Input: part model. Units: mm. Frame: model coordinates. A direction names the side the tool comes from. Coordinates: 2 decimals unless noted, no trailing zeros. Order: outer loops, then holes, each group sorted by start corner. A loop starts at its lowest first (then second) coordinate and runs counter-clockwise, first axis right, second up.
Autodesk Inventor part; units mm, degrees
ref_plane "Work Plane2" through (-37, -48, -28.5) normal (0, 0, 1) x (1, 0, 0)
ref_plane "YZ Plane" through (0, 0, 0) normal (1, 0, 0) x (0, 1, 0)
ref_plane "XZ Plane" through (0, 0, 0) normal (0, 1, 0) x (-1, 0, 0)
ref_plane "Work Plane1" through (0, 0, 0) normal (0, 0, 1) x (1, 0, 0)
sketch "Sketch1" plane through (0, 0, 0) normal (0, 0, 1) x (1, 0, 0)
  arc A0 (27, -22.0618) -> (22.0618, -27) centre (24.7, -24.7) ccw construction
  line L0 (27, 0) -> (27, -22.0618) construction
  line L1 (27, 0) -> (0, 0) construction
  line L2 (0, 0) -> (0, -27) construction
  line L3 (22.0618, -27) -> (0, -27) construction
  circle A1 centre (13, -13) radius 1.65 construction
  circle A2 centre (10, -22.5) radius 1.55 construction
  circle A3 centre (10, -7.5) radius 1.55 construction
  circle A4 centre (20, -20) radius 1.05 construction
  circle A5 centre (7.5, -10) radius 1.55 construction
  circle A6 centre (22.5, -10) radius 1.55 construction
  arc A7 (22.0618, -33) -> (27, -37.9382) centre (24.7, -35.3) ccw construction
  line L4 (0, -33) -> (22.0618, -33) construction
  line L5 (0, -33) -> (0, -60) construction
  line L6 (0, -60) -> (27, -60) construction
  line L7 (27, -37.9382) -> (27, -60) construction
  circle A8 centre (13, -47) radius 1.65 construction
  circle A9 centre (10, -52.5) radius 1.55 construction
  circle A10 centre (10, -37.5) radius 1.55 construction
  circle A11 centre (20, -40) radius 1.05 construction
  circle A12 centre (7.5, -50) radius 1.55 construction
  circle A13 centre (22.5, -50) radius 1.55 construction
  arc A14 (33, -37.9382) -> (37.9382, -33) centre (35.3, -35.3) ccw construction
  line L8 (33, -60) -> (33, -37.9382) construction
  line L9 (33, -60) -> (60, -60) construction
  line L10 (60, -60) -> (60, -33) construction
  line L11 (37.9382, -33) -> (60, -33) construction
  circle A15 centre (47, -47) radius 1.65 construction
  circle A16 centre (50, -52.5) radius 1.55 construction
  circle A17 centre (50, -37.5) radius 1.55 construction
  circle A18 centre (40, -40) radius 1.05 construction
  circle A19 centre (37.5, -50) radius 1.55 construction
  circle A20 centre (52.5, -50) radius 1.55 construction
  arc A21 (37.9382, -27) -> (33, -22.0618) centre (35.3, -24.7) ccw construction
  line L12 (60, -27) -> (37.9382, -27) construction
  line L13 (60, -27) -> (60, 0) construction
  line L14 (60, 0) -> (33, 0) construction
  line L15 (33, -22.0618) -> (33, 0) construction
  circle A22 centre (47, -13) radius 1.65 construction
  circle A23 centre (50, -22.5) radius 1.55 construction
  circle A24 centre (50, -7.5) radius 1.55 construction
  circle A25 centre (40, -20) radius 1.05 construction
  circle A26 centre (37.5, -10) radius 1.55 construction
  circle A27 centre (52.5, -10) radius 1.55 construction
  line L16 (60, 0) -> (-37, 0) construction
  line L17 (-37, 0) -> (-37, -60) construction
  line L18 (-37, -60) -> (60, -60) construction
  line L19 (60, -60) -> (60, 0) construction
  line L20 (60, 0) -> (-37, 0)
  line L21 (-37, 0) -> (-37, -60)
  line L22 (-37, -60) -> (60, -60)
  line L23 (60, -60) -> (60, 0)
  line L24 (-37, 0) -> (-37, -48)
extrude "Extrusion1" add sketch "Sketch1" along normal blind 10
sketch "Sketch2" plane through (0, 0, 0) normal (0, 0, -1) x (-1, 0, 0)
  circle A0 centre (21, -3) radius 1
  circle A1 centre (28.5, -33) radius 1
  circle A2 centre (12.5, -33) radius 1.0474
  circle A3 centre (12.5, -43) radius 1
  circle A4 centre (21, -43) radius 1
  circle A5 centre (28.5, -43) radius 1
  circle A6 centre (21, -33) radius 1
  circle A7 centre (29, -3) radius 1
  circle A8 centre (13, -3) radius 1
  line L0 (37, 0) -> (5, 0)
  line L1 (37, 0) -> (37, -48)
  line L2 (5, -48) -> (37, -48)
  line L3 (5, 0) -> (5, -48)
  line L4 (37, -48) -> (5, -48)
  line L5 (5, -48) -> (5, -60)
  line L6 (5, -60) -> (37, -60)
  line L7 (37, -60) -> (37, -48)
  point P0 (0, 0)
ref_plane "Work Plane2" through (-37, -48, -28.5) normal (0, 0, 1) x (1, 0, 0)
extrude "Extrusion2" add sketch "Sketch2" along normal up to surface (28.5 mm away) contours A0 | A1 | A2 | A3 | A4 | A5 | A6 | A7 | A8 | L1 L2 L3 L0 | L7 L6 L5 L2
sketch "Sketch3" plane through (0, 0, 10) normal (0, 0, 1) x (1, 0, 0)
  line L0 (0, 0) -> (0, -60) construction
  line L1 (60, 0) -> (0, 0) construction
  line L2 (60, -60) -> (60, 0) construction
  line L3 (0, -60) -> (60, -60) construction
  line L4 (27.1959, -58) -> (26.6538, -58) construction
  line L5 (27.7692, -53.6731) -> (27.1959, -58) construction
  line L6 (29.9435, -58) -> (27.7692, -53.6731) construction
  line L7 (30.0649, -58) -> (29.9435, -58) construction
  line L8 (32.2308, -53.6827) -> (30.0649, -58) construction
  line L9 (32.8053, -58) -> (32.2308, -53.6827) construction
  line L10 (33.3462, -58) -> (32.8053, -58) construction
  line L11 (32.5493, -52) -> (33.3462, -58) construction
  line L12 (32.4712, -52) -> (32.5493, -52) construction
  line L13 (30, -56.9231) -> (32.4712, -52) construction
  line L14 (27.5228, -52) -> (30, -56.9231) construction
  line L15 (27.4459, -52) -> (27.5228, -52) construction
  line L16 (26.6538, -58) -> (27.4459, -52) construction
  circle A0 centre (24.7, -24.7) radius 1.6 construction
  circle A1 centre (35.3, -24.7) radius 1.6 construction
  circle A2 centre (35.3, -35.3) radius 1.6 construction
  circle A3 centre (24.7, -35.3) radius 1.6 construction
  circle A4 centre (52.5, -50) radius 1.55 construction
  circle A5 centre (52.5, -10) radius 1.55 construction
  circle A6 centre (37.5, -50) radius 1.55 construction
  circle A7 centre (37.5, -10) radius 1.55 construction
  circle A8 centre (22.5, -50) radius 1.55 construction
  circle A9 centre (22.5, -10) radius 1.55 construction
  circle A10 centre (7.5, -50) radius 1.55 construction
  circle A11 centre (7.5, -10) radius 1.55 construction
  circle A12 centre (40, -40) radius 1.05 construction
  circle A13 centre (20, -40) radius 1.05 construction
  circle A14 centre (40, -20) radius 1.05 construction
  circle A15 centre (20, -20) radius 1.05 construction
  circle A16 centre (47, -47) radius 1.65 construction
  circle A17 centre (13, -47) radius 1.65 construction
  circle A18 centre (30, -47) radius 1.65 construction
  circle A19 centre (47, -13) radius 1.65 construction
  circle A20 centre (13, -13) radius 1.65 construction
  circle A21 centre (30, -13) radius 1.65 construction
  circle A22 centre (47, -30) radius 1.65 construction
  circle A23 centre (13, -30) radius 1.65 construction
  circle A24 centre (30, -30) radius 1.65 construction
  circle A25 centre (10, -52.5) radius 1.55 construction
  circle A26 centre (10, -37.5) radius 1.55 construction
  circle A27 centre (10, -22.5) radius 1.55 construction
  circle A28 centre (10, -7.5) radius 1.55 construction
  circle A29 centre (50, -52.5) radius 1.55 construction
  circle A30 centre (50, -37.5) radius 1.55 construction
  circle A31 centre (50, -22.5) radius 1.55 construction
  circle A32 centre (50, -7.5) radius 1.55 construction
  circle A33 centre (13, -13) radius 1.65 construction
  circle A34 centre (13, -13) radius 1.65
  circle A35 centre (47, -13) radius 1.65
  circle A36 centre (47, -47) radius 1.65
  circle A37 centre (13, -47) radius 1.65
  circle A38 centre (13, -13) radius 2
  circle A39 centre (47, -13) radius 2
  circle A40 centre (47, -47) radius 2
  circle A41 centre (13, -47) radius 2
  dimension "d6" = 4
  dimension "d7" = 4
  dimension "d8" = 4
  dimension "d9" = 4
extrude "Extrusion3" cut sketch "Sketch3" against normal through all contours A34 | A35 | A36 | A37 | A38 | A39 | A40 | A41
sketch "Sketch4" plane through (0, 0, 10) normal (0, 0, 1) x (1, 0, 0)
  circle A0 centre (-21, -3) radius 1
  circle A1 centre (-28.5, -33) radius 1
  circle A2 centre (-12.5, -33) radius 1.0474
  circle A3 centre (-12.5, -43) radius 1
  circle A4 centre (-21, -43) radius 1
  circle A5 centre (-28.5, -43) radius 1
  circle A6 centre (-21, -33) radius 1
  circle A7 centre (-29, -3) radius 1
  circle A8 centre (-13, -3) radius 1
  line L0 (-37, 0) -> (-5, 0)
  line L1 (-37, 0) -> (-37, -48)
  line L2 (-5, -48) -> (-37, -48)
  line L3 (-5, 0) -> (-5, -48)
  point P0 (0, 0)
hole "Hole1" at (-12.5, -43, 10) at (-21, -43, 10) at (-28.5, -43, 10) at (-28.5, -33, 10) at (-21, -33, 10) at (-12.5, -33, 10) at (-13, -3, 10) at (-21, -3, 10) at (-29, -3, 10) direction (0, 0, -1) diameter 3.5 end through all counterbore diameter 7 counterbore depth 30
sketch "Sketch5" plane through (-37, -60, 10) normal (0, -1, 0) x (1, 0, 0)
  line L0 (32, -10) -> (97, -10)
  line L1 (97, -10) -> (97, 0)
  line L2 (0, 0) -> (97, 0)
  line L3 (0, -38.5) -> (0, 0)
  line L4 (32, -38.5) -> (0, -38.5)
  line L5 (32, -10) -> (32, -38.5)
  circle A0 centre (16, -54.5) radius 2.5 construction
  line L6 (0, -70.5) -> (32, -70.5)
  line L7 (32, -38.5) -> (0, -38.5)
  line L8 (0, -38.5) -> (0, -70.5)
  line L9 (0, -70.5) -> (32, -70.5)
  line L10 (32, -70.5) -> (32, -38.5)
  circle A1 centre (16, -54.5) radius 12.5
  point P0 (37, -10)
  dimension "d18" = 25
extrude "Extrusion4" add sketch "Sketch5" against normal blind 10 contours L10 L6 L8 L4
sketch "Sketch6" plane through (-37, -60, 10) normal (0, -1, 0) x (1, 0, 0)
  circle A0 centre (16, -54.5) radius 12.5
  arc A1 (22.2144, -58.2891) -> (16.4089, -42.0067) centre (9.2362, -53.7403) ccw
  circle A2 centre (16, -54.5) radius 12.5
  arc A3 (20.9144, -57.4347) -> (13.4909, -42.2544) centre (9.2362, -53.7403) ccw
  line L0 (22.2144, -58.2891) -> (20.9144, -57.4347)
  arc A4 (16.4089, -42.0067) -> (13.4909, -42.2544) centre (16, -54.5) ccw
  point P0 (37, -10)
  dimension "d21" = 1.3
extrude "Extrusion5" add sketch "Sketch6" against normal up to surface (10 mm away) contours A1 L0 A3 A0 picked at (20.8673, -47.5497)
pattern_circular "Circular Pattern1" count 3 over 360 about axis through (-21, -60, -44.5) along (0, 1, 0) of "Extrusion5"
sketch "Sketch7" plane through (-37, -60, 10) normal (0, -1, 0) x (1, 0, 0)
  arc A0 (27.8595, -58.4499) -> (16.4089, -42.0067) centre (16, -54.5) ccw
  line L0 (3, -41.5) -> (29, -41.5) construction
  line L1 (29, -41.5) -> (29, -67.5) construction
  line L2 (29, -67.5) -> (3, -67.5) construction
  line L3 (3, -67.5) -> (3, -41.5) construction
  line L4 (3, -41.5) -> (29, -67.5) construction
  line L5 (29, -41.5) -> (3, -67.5) construction
  line L6 (16, -54.5) -> (16, -34.5) construction
  point P0 (37, -10)
  dimension "d27" = 26
  dimension "d28" = 26
  dimension "d29" = 20
hole "Hole2" at (-8, -60, -57.5) at (-34, -60, -57.5) at (-21, -60, -24.5) direction (0, 1, 0) diameter 2.9 depth 10 tip angle 118 counterbore diameter 6 counterbore depth 4
properties part number "04_Bridge_Laser_Nanomax"
Item 1: Cut plane D-D on y = -24.5. Return loops of the section in (x, z).
Response values:
outline: (-37, -28.5) - (-5, -28.5) - (-5, 0) - (60, 0) - (60, 10) - (-37, 10) - close
Item 2: Ray query, probe 1 along X at (y, z) = (-3, -2); probe 2 along X at (y, z) = (-43, -10); probe 3 along Y at (x, z) = (-21, -26). Return the intervals inside material, ascending.
Response values:
probe 1: x = -37 to -32.5, -25.5 to -24.5, -17.5 to -16.5, -9.5 to -5
probe 2: x = -37 to -32, -25 to -24.5, -17.5 to -16, -9 to -5
probe 3: y = -56 to -44.75, -41.25 to -34.75, -31.25 to -4.75, -1.25 to 0
Item 3: Cut plane B-B on y = -33. Count the separate pieces of the cut face and the enclosed holes in it, then the cut area to 3 significant figures.
Response values:
separate pieces: 4
enclosed holes: 0
area: 1,160 mm2
Item 4: Draft query along Z for faces 5 (the face through (27, -30, 0)), 6 (the face through (-8.06, -52.96, -56.05)), 7 (the face through (-14.735, -2.772, -24.31)). Return one class per face: pulls with the +Z half, pulls with the -Z half, needs draft (parallel to the pull), parting line crosses it, or undercut.
Response values:
face 5: pulls with the -Z half
face 6: undercut
face 7: needs draft
Item 5: Access query for faces 1 (the face through (-24.47, -32.54, -5.21)), 2 (the face through (-21, -50, -51)), 3 (the face through (-28.364, -55.07, -43.791)), 4 (the face through (-21.1, -58, -21.5)). Directions: +Z, -Z, +X, -X, +Y, -Y. A direction counts if a zero-diameter tool reaches every point of the face in a straight line with its end or side. Return the directions, or none.
Response values:
face 1: +Z
face 2: -Z, +X, -X, +Y
face 3: +Y, -Y
face 4: -Y
Item 6: Cut plane A-A on x = 13. Return loops of the section in (y, z), then the cut area to 3 significant figures.
Response values:
outline: (-60, 0) - (-49, 0) - (-49, 10) - (-60, 10) - close; (-45, 0) - (-15, 0) - (-15, 10) - (-45, 10) - close; (-11, 0) - (0, 0) - (0, 10) - (-11, 10) - close
area: 520 mm2
Item 7: Pin query (flat end, axial travel): pin 1 Ø5 at (x, y) = (-10, -45) entering from -Z; pin 2 Ø7 at (x, y) = (-28, -2.5) entering from +Z; pin 3 Ø8 at (x, y) = (45, -36) entering from -Z; pin 4 Ø6.5 at (x, y) = (-21, -43) entering from +Z. Return the tip coordinate at first contact, or that it passes through.
Response values:
pin 1: stops at z = -28.5
pin 2: stops at z = 10
pin 3: stops at z = 0
pin 4: stops at z = -20
